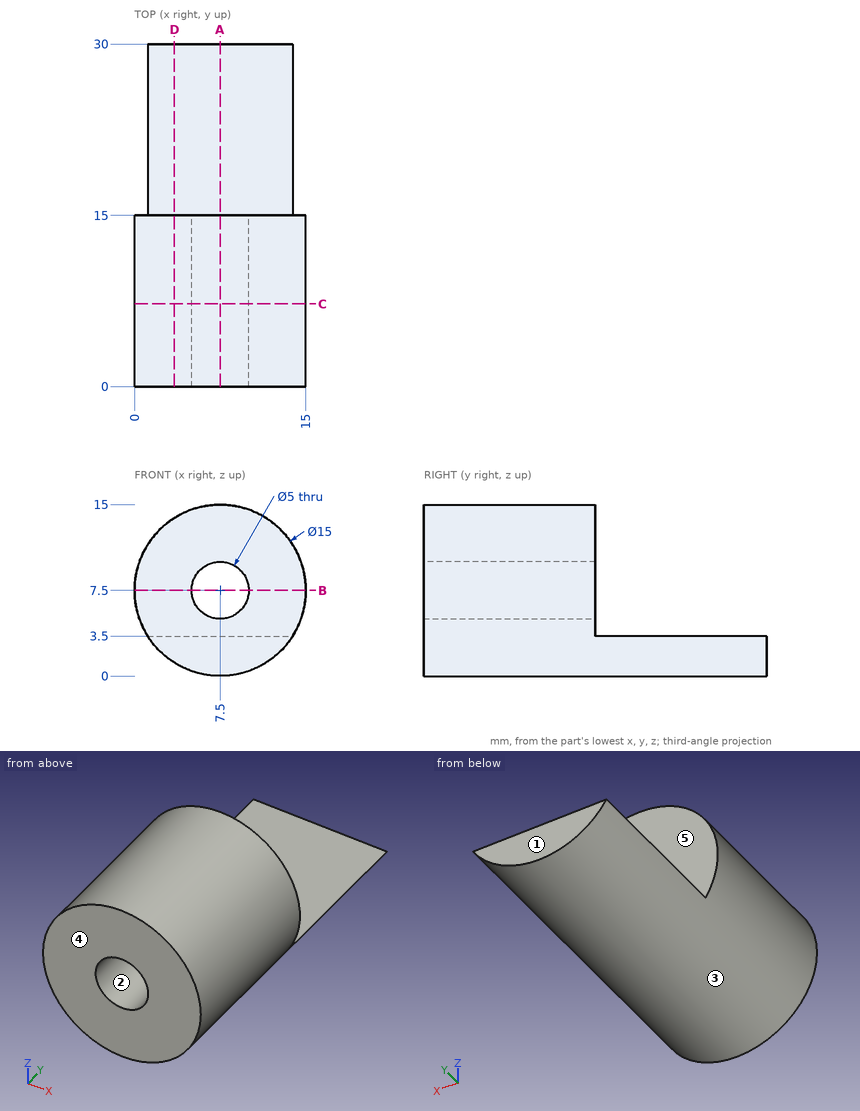
Answer from the drawing. Dimensions are ordinates in mm from the lowest x, y and z of the part. A direction names the side the tool comes from. Give positions to 0.01 mm unless a question says otherwise; leave off trailing zeros. Order: outer loops, then holes, each group sorted by start corner. A loop starts at its lowest first (then second) coordinate and runs counter-clockwise, first axis right, second up. Notation, with made-up numbers: (17, 44) - (22, 44) arc R16 ccw to (22, 73) - close; hole circle Ø11 at (68, -5). An arc over 180 degrees is marked (long way). Use one line per item in the form item = value.
1) Find section C-C on y = 7.25. Determine the outline of the cut face in (x, z).
Verdict:
outline = circle Ø15 at (7.5, 7.5); hole circle Ø5 at (7.5, 7.5)
2) Each of these flat-tipped pins is pushed along its axis until it touches: pin 1 (1.5 mm diameter, centred on x = 6, y = 15.5, fed in from -Z); pin 2 (3.5 mm diameter, centred on x = 10, z = 7.5, fed in from +Y); pin 3 (2 mm diameter, centred on y = 20, z = 1.5, fed in from +X); pin 4 (3 mm diameter, centred on x = 7.5, z = 7.5, fed in from +Y). Where does it stop, or does it pass through?
Verdict:
pin_1 = 0.04
pin_2 = 15
pin_3 = 13.09
pin_4 = through
3) The mould has two halves that part along X. Classify the marked faces 1, 2 and 3: released by +X, released by -X, zero draft, split by the parting line, or undercut.
Verdict:
face_1 = zero draft
face_2 = undercut
face_3 = split by the parting line
4) Find section B-B on z = 7.5. Determine the outline of the cut face in (x, y), and give its area (3 significant figures).
Verdict:
outline = (0, 0) - (5, 0) - (5, 15) - (0, 15) - close; (10, 0) - (15, 0) - (15, 15) - (10, 15) - close
area = 150 mm^2
5) Find section D-D on x = 3.5. Determine the outline of the cut face in (y, z).
Verdict:
outline = (0, 1.16) - (30, 1.16) - (30, 3.5) - (15, 3.5) - (15, 13.84) - (0, 13.84) - close
6) Find section A-A on x = 7.5. Determine the outline of the cut face in (y, z).
Verdict:
outline = (0, 0) - (30, 0) - (30, 3.5) - (15, 3.5) - (15, 5) - (0, 5) - close; (0, 10) - (15, 10) - (15, 15) - (0, 15) - close
7) For the marked faces 4 and 5, determine the directions among +Z, -Z, +X, -X, +Y, -Y from which every point of the face is accessible in a straight line to the end or side of a thin tool.
Verdict:
face_4 = +Z, -Z, +X, -X, -Y
face_5 = +Z, +X, -X, +Y
8) Consider probe 1 along X at (y, z) = (11, 7.5); probe 2 along Y at (x, z) = (3, 10.5); probe 3 along Z at (x, y) = (11.5, 28.25). Determine where each line is inside the solid, lowest interval first. Write a range as [from, to].
Verdict:
probe_1 = [0, 5], [10, 15]
probe_2 = [0, 15]
probe_3 = [1.16, 3.5]
